Could you check a few things on this model? Use its own coordinates, in mm. Face numbers are marked on the shaded views. A direction names the side the tool comes from. Coordinates: 2 decimals unless noted, no trailing zeros. Loops run counter-clockwise (first coordinate to the right, second up) from the corner with the lowest first, then second, coordinate; pieces in that order, holes last. Notation, with made-up numbers: (19.5, -16) -> (63.5, -16) arc R14 ccw to (63.5, -8) -> close; hole circle Ø7 at (47, -19). An arc over 180 degrees is marked (long way). One line per question, with ' | ' between items.
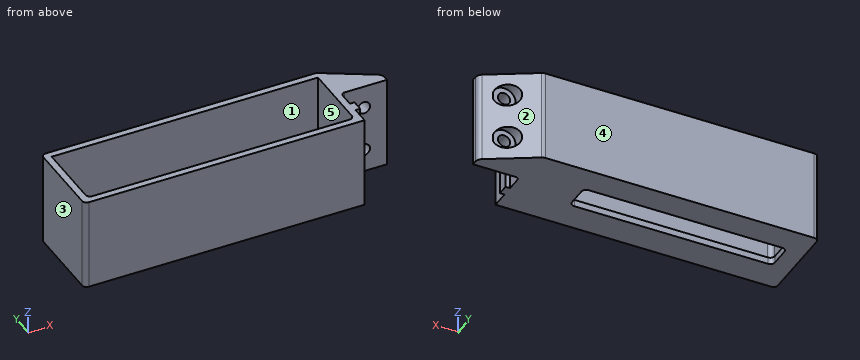
```python
from build123d import *

# Parameters (mm, degrees)
SKETCH1_W                      = 115.5
SKETCH1_H                      = 30.5
SKETCH1_W_2                    = 88
SKETCH1_H_2                    = 12
BOSS_EXTRUDE1_DEPTH            = 3
BOSS_EXTRUDE2_START            = 37
SKETCH1_3_W                    = 115.5
SKETCH1_3_H                    = 30.5
BOSS_EXTRUDE2_DEPTH            = 37
CBORE_FOR_M5_SHCS1_D           = 5.3
CBORE_FOR_M5_SHCS1_CBORE_D     = 10
CBORE_FOR_M5_SHCS1_CBORE_DEPTH = 9.75
FILLET1_R                      = 2
FILLET2_R                      = 1.5


with BuildPart() as part:
    # Sketch1 → Boss-Extrude1 (new body)
    # profile 1 of 2: a face of its own
    with BuildSketch(Plane.XY):
        with BuildLine():
            Line((23, 17), (23, 19))
            ThreePointArc((23, 19), (22.596751829, 20.502291563), (21.495413373, 21.600718909))
            Line((21.495413373, 21.600718909), (1.495413373, 33.100718909))
            ThreePointArc((1.495413373, 33.100718909), (0.773900275, 33.398461379), (0, 33.5))
            Line((0, 33.5), (-118.5, 33.5))
            Line((-118.5, 33.5), (-118.5, -3))
            Line((-118.5, -3), (3, -3))
            Line((3, -3), (3, 4.6))
            Line((3, 4.6), (5, 4.6))
            Line((5, 4.6), (5, 9.4))
            Line((5, 9.4), (3, 9.4))
            Line((3, 9.4), (3, 17))
            Line((3, 17), (23, 17))
        make_face()
        with Locations((-57.75, 15.25)):
            Rectangle(SKETCH1_W, SKETCH1_H, mode=Mode.SUBTRACT)
    # profile 2 of 2: a face of its own
    with BuildSketch(Plane.XY):
        with Locations((-57.75, 15.25)):
            Rectangle(SKETCH1_W, SKETCH1_H)
        with Locations((-66.5, 16)):
            Rectangle(SKETCH1_W_2, SKETCH1_H_2, mode=Mode.SUBTRACT)
    extrude(amount=-BOSS_EXTRUDE1_DEPTH)

    # Sketch1<3> → Boss-Extrude2 (add)
    with BuildSketch(Plane.XY.offset(BOSS_EXTRUDE2_START)):
        with BuildLine():
            Line((23, 17), (23, 19))
            ThreePointArc((23, 19), (22.596751829, 20.502291563), (21.495413373, 21.600718909))
            Line((21.495413373, 21.600718909), (1.495413373, 33.100718909))
            ThreePointArc((1.495413373, 33.100718909), (0.773900275, 33.398461379), (0, 33.5))
            Line((0, 33.5), (-118.5, 33.5))
            Line((-118.5, 33.5), (-118.5, -3))
            Line((-118.5, -3), (3, -3))
            Line((3, -3), (3, 4.6))
            Line((3, 4.6), (5, 4.6))
            Line((5, 4.6), (5, 9.4))
            Line((5, 9.4), (3, 9.4))
            Line((3, 9.4), (3, 17))
            Line((3, 17), (23, 17))
        make_face()
        with Locations((-57.75, 15.25)):
            Rectangle(SKETCH1_3_W, SKETCH1_3_H, mode=Mode.SUBTRACT)
    extrude(amount=-BOSS_EXTRUDE2_DEPTH)

    # CBORE for M5 SHCS1 (through all)
    with Locations(Plane(origin=(0, 33.5, 0), x_dir=(1, 0, 0), z_dir=(0, 1, 0))):
        with Locations((13, -27), (13, -7)):
            CounterBoreHole(CBORE_FOR_M5_SHCS1_D / 2, CBORE_FOR_M5_SHCS1_CBORE_D / 2, CBORE_FOR_M5_SHCS1_CBORE_DEPTH)

    # Fillet1
    fillet1_edges = [part.edges().sort_by_distance(p)[0] for p in [
        (-22.5, 22, -1.5),
        (-110.5, 22, -1.5),
        (-110.5, 10, -1.5),
        (-22.5, 10, -1.5),
        (-118.5, -3, 17),
        (-118.5, 33.5, 17),
        (0, 0, 18.5),
        (-57.75, 0, 0),
        (-115.5, 0, 18.5),
    ]]
    fillet(fillet1_edges, radius=FILLET1_R)

    # Fillet2
    fillet2_edges = [part.edges().sort_by_distance(p)[0] for p in [
        (3, 17, 17),
    ]]
    fillet(fillet2_edges, radius=FILLET2_R)


solid = part.part
```
Q1. Imagine slicing it at A-A on z = 7. Give the number of separate pieces and of enclosed holes in the cut face, plus the area to 3 significant figures.
Values follow:
separate pieces: 2 | enclosed holes: 1 | area: 1,050 mm2
Q2. For pin 1 (9 mm diameter, centred on x = 17.5, z = 13.5, fed in from -Y); pin 2 (12 mm diameter, centred on y = 27, z = 15.5, fed in from +X); pin 3 (0.6 mm diameter, centred on x = 4, z = 9, fed in from +Y), each with a flat end and sliding along its axis, tell me the tip position at first contact or that it passes through.
Values follow:
pin 1: stops at y = 17 | pin 2: stops at x = 22.24 | pin 3: stops at y = 31.83
Q3. Please list where these lines run through material, in increasing order: L1, parallel to Z at x = 13, y = 25; L2, parallel to Z at x = 13, y = 18.5; L3, parallel to Y at x = -11.5, z = 6.5. Write a range as [from, to].
Values follow:
L1: z = [-3, 2], [12, 22], [32, 37] | L2: z = [-3, 4.35], [9.65, 24.35], [29.65, 37] | L3: y = [-3, 0], [30.5, 33.5]
Q4. Imagine slicing it at C-C on z = 13.5. Write out the boundary of the cut face in (x, y), plus the area to 3 significant figures.
Values follow:
outline: (-118.5, -1) arc R2 ccw to (-116.5, -3) -> (3, -3) -> (3, 4.6) -> (5, 4.6) -> (5, 9.4) -> (3, 9.4) -> (3, 15.5) arc R1.5 cw to (4.5, 17) -> (23, 17) -> (23, 19) arc R3 ccw to (21.5, 21.6) -> (1.5, 33.1) arc R3 ccw to (0, 33.5) -> (-116.5, 33.5) arc R2 ccw to (-118.5, 31.5) -> close; hole (-115.5, 2) arc R2 ccw to (-113.5, 0) -> (-2, 0) arc R2 ccw to (0, 2) -> (0, 30.5) -> (-115.5, 30.5) -> close | area: 1,110 mm2
Q5. For the marked faces 4 and 5, which set-ups out of +Z, -Z, +X, -X, +Y, -Y let a thin tool reach every point of the face, with its end or its side?
Values follow:
face 4: +Z, -Z, +X, -X, +Y | face 5: +Z
Q6. Imagine slicing it at B-B on y = 8. Write out the boundary of the cut face in (x, z).
Values follow:
outline: (-118.5, -3) -> (5, -3) -> (5, 37) -> (0, 37) -> (0, 0) -> (-115.5, 0) -> (-115.5, 37) -> (-118.5, 37) -> close
Q7. Imagine slicing it at D-D on x = 13. Write out the boundary of the cut face in (y, z), plus the area to 3 significant figures.
Values follow:
outline: (17, -3) -> (26.49, -3) -> (26.49, 2) -> (23.75, 2) -> (23.75, 4.35) -> (17, 4.35) -> close; (17, 9.65) -> (23.75, 9.65) -> (23.75, 12) -> (26.49, 12) -> (26.49, 22) -> (23.75, 22) -> (23.75, 24.35) -> (17, 24.35) -> close; (17, 29.65) -> (23.75, 29.65) -> (23.75, 32) -> (26.49, 32) -> (26.49, 37) -> (17, 37) -> close | area: 253 mm2
Q8. We'd pull the mould along X, two halves only. Please class the marked faces 1, 2 and 3: released by +X, released by -X, zero draft, split by the parting line, or undercut.
Values follow:
face 1: undercut | face 2: released by +X | face 3: released by -X
